Geometry check sheet. Reference: drawing and pictorial views, mm from the part's lowest x, y, z. Coordinates: 2 decimals unless noted, no trailing zeros. Loops run counter-clockwise (first coordinate to the right, second up) from the corner with the lowest first, then second, coordinate; pieces in that order, holes last. Notation, with made-up numbers: (74.25, -28) - (95.25, -28) arc R24 ccw to (95.25, -3) - close; hole circle Ø4 at (21, 7). An arc over 180 degrees is marked (long way). Use a Markdown table: item, result. Add a question column.
1) Go/stop test with flat-tipped pins: P1, Ø11.5, axis at x = 68.58, y = 7.62, coming from the -Z side; P2, Ø1, axis at y = 20.5, z = 31, coming from the +X side; P3, Ø4, axis at y = 10, z = 30, coming from the -X side; P4, Ø4, axis at x = 14.5, y = 4, coming from the +Z side. Record where each tip stops, or that it passes through.
2) Draft check along X on the marked faces 1, 2, 3 and 4. Enter one of: pulls with the +X half, pulls with the -X half, needs draft (parallel to the pull), parting line crosses it, or undercut.
3) Sectioned sample at B-B, the plane z = 21.5. Enter the section's corners in (x, y), then the cut area to 3 significant figures.
4) Sectioned sample at C-C, the plane y = 30.48. Enter the section's corners in (x, z).
5) Thickness scan on line 1 (Y direction, x = 7.62, z = 16); line 2 (X direction, y = 8, z = 8.5); line 3 (X direction, y = 7, z = 11). Record the ranges inside material, lowest first.
6) Sectioned sample at A-A, the plane x = 68.58. Enter the section's corners in (y, z).
7) Sectioned sample at D-D, the plane x = 5. Enter the section's corners in (y, z) (1 decimal), then the cut area to 3 significant figures.
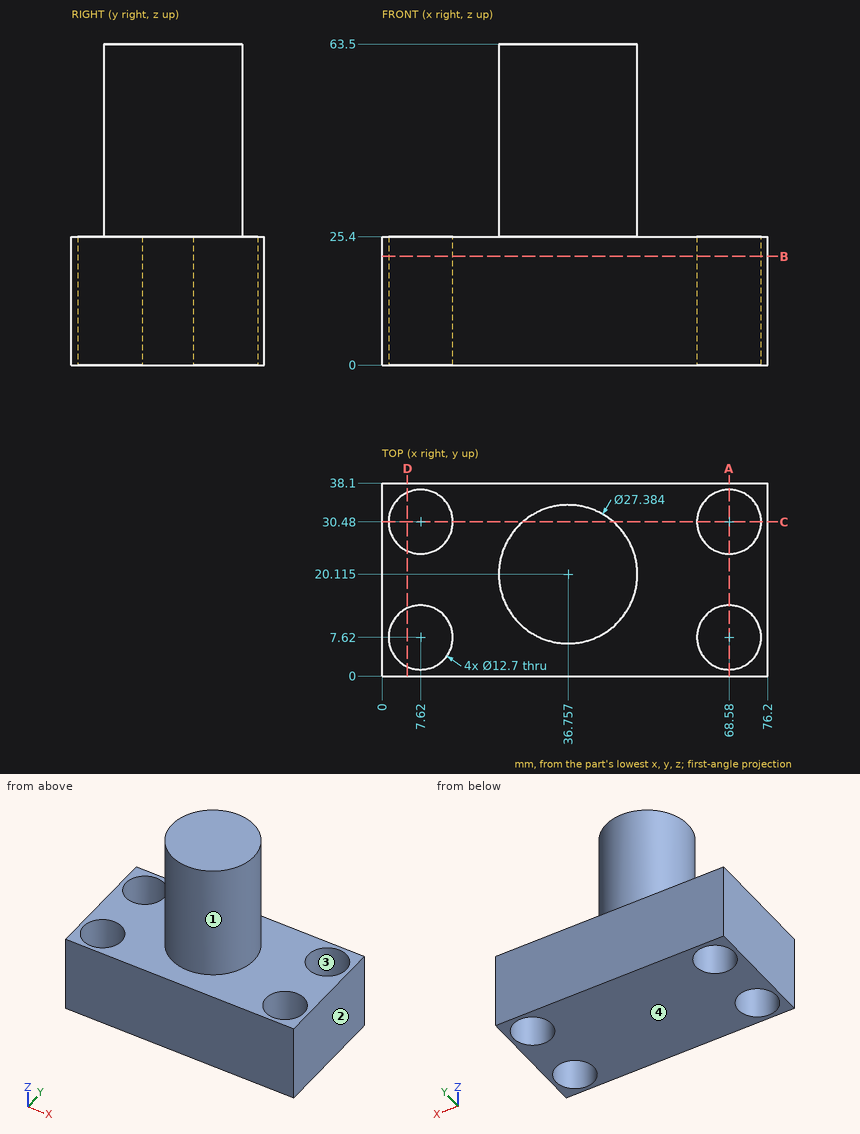
Solved:
| question | item | result |
|---|---|---|
| 1 | P1 | passes through |
| 1 | P2 | stops at x = 50.45 |
| 1 | P3 | stops at x = 25.73 |
| 1 | P4 | stops at z = 25.4 |
| 2 | face 1 | parting line crosses it |
| 2 | face 2 | pulls with the +X half |
| 2 | face 3 | undercut |
| 2 | face 4 | needs draft |
| 3 | outline | (0, 0) - (76.2, 0) - (76.2, 38.1) - (0, 38.1) - close; hole circle Ø12.7 at (7.62, 7.62); hole circle Ø12.7 at (7.62, 30.48); hole circle Ø12.7 at (68.58, 7.62); hole circle Ø12.7 at (68.58, 30.48) |
| 3 | area | 2,400 mm2 |
| 4 | outline | (0, 0) - (1.27, 0) - (1.27, 25.4) - (0, 25.4) - close; (13.97, 0) - (62.23, 0) - (62.23, 25.4) - (45.7, 25.4) - (45.7, 63.5) - (27.81, 63.5) - (27.81, 25.4) - (13.97, 25.4) - close; (74.93, 0) - (76.2, 0) - (76.2, 25.4) - (74.93, 25.4) - close |
| 5 | line 1 | y = 0 to 1.27, 13.97 to 24.13, 36.83 to 38.1 |
| 5 | line 2 | x = 0 to 1.28, 13.96 to 62.24, 74.92 to 76.2 |
| 5 | line 3 | x = 0 to 1.3, 13.94 to 62.26, 74.9 to 76.2 |
| 6 | outline | (0, 0) - (1.27, 0) - (1.27, 25.4) - (0, 25.4) - close; (13.97, 0) - (24.13, 0) - (24.13, 25.4) - (13.97, 25.4) - close; (36.83, 0) - (38.1, 0) - (38.1, 25.4) - (36.83, 25.4) - close |
| 7 | outline | (0, 0) - (1.8, 0) - (1.8, 25.4) - (0, 25.4) - close; (13.4, 0) - (24.7, 0) - (24.7, 25.4) - (13.4, 25.4) - close; (36.3, 0) - (38.1, 0) - (38.1, 25.4) - (36.3, 25.4) - close |
| 7 | area | 380 mm2 |
